Source: CAD feature listing. Evaluate the final solid. Frame: model axes, mm. A direction names the side the tool comes from. Give positions to 0.01 mm unless a question says otherwise; leave off trailing zeros. Write each loop counter-clockwise with the first axis right and the second up, starting at its lowest first coordinate (ties: lowest second). Pieces come first, ordered by that corner, then holes. Notation, with made-up numbers: (37.25, 77) -> (73.25, 77) arc R12 cw to (73.25, 98) -> close; hole circle Ø3 at (0, -37.5). An arc over 180 degrees is marked (long way). Use one line per item in the form item = value. Start each with the question number.
(1) Cut plane A-A, the plane z = 877. Output: boundary loops of the cut face in (x, y), and give its area (3 significant figures).
(2) Draft query along Z for faces 1 (the face through (71.048, -41.672, 776.376)), 2 (the face through (56, -61, 1574.8)), 3 (the face through (101.6, -169, 776)). Return one class per face: pulls with the +Z half, pulls with the -Z half, needs draft (parallel to the pull), parting line crosses it, or undercut.
(3) Material intervals for line 1 along Z through (x, y) = (8, -58); line 2 along Y through (x, z) = (25.4, 9.5); line 3 along X through (y, z) = (-198, 274), sorted ascending. Write a range as from..to.
(4) First-contact query: P1, Ø20.5, axis at x = 45.5, z = 8.5, coming from the -Y side; P2, Ø3, axis at x = 86, z = 1276.5, coming from the -Y side; P3, Ø5, axis at x = 13, z = 962, coming from the -Y side. Flat tips, straight axial feed; report the tip coordinate or a pass-through.
(5) Set-up query: faces 4 (the face through (114.3, -164, 776)), 5 (the face through (48, -88.032, 13)), 6 (the face through (48, -58, 25.4)). Return all of +Z, -Z, +X, -X, +Y, -Y with unobstructed straight access to the full face (end or side cutting, diameter ignored); none if empty.
from build123d import *

# Parameters (mm, degrees)
BOSS_EXTRUDE1_DEPTH = 1574.8
BOSS_EXTRUDE2_DEPTH = 25.4
SKETCH3_R           = 19.05
CUT_EXTRUDE1_DEPTH  = 1575.8


with BuildPart() as part:
    # Sketch1 → Boss-Extrude1 (new body)
    with BuildSketch(Plane.XY):
        with BuildLine():
            ThreePointArc((114.3, -101.6), (84.542048969, -29.757951031), (12.7, 0))
            ThreePointArc((12.7, 0), (6.337512086, -0.199414462), (0, -0.796875048))
            Line((0, -0.796875048), (0, -12.7))
            ThreePointArc((0, -12.7), (71.842048969, -42.457951031), (101.6, -114.3))
            Line((101.6, -114.3), (101.6, -224.550826558))
            Line((101.6, -224.550826558), (114.3, -224.550826558))
            Line((114.3, -224.550826558), (114.3, -101.6))
        make_face()
    extrude(amount=BOSS_EXTRUDE1_DEPTH)

    # Sketch2 → Boss-Extrude2 (add)
    with BuildSketch(Plane(origin=(0, 0, 0), x_dir=(-1, 0, 0), z_dir=(0, 0, -1))):
        with BuildLine():
            Line((0, -0.796875048), (0, -88.032487207))
            Line((0, -88.032487207), (-113.39003226, -88.032487207))
            ThreePointArc((-113.39003226, -88.032487207), (-74.652194888, -21.073696542), (0, -0.796875048))
        make_face()
    boss_extrude2 = extrude(amount=-BOSS_EXTRUDE2_DEPTH)

    # Mirror2: Boss-Extrude2 across plane
    add(boss_extrude2.mirror(Plane(origin=(0, 0, 787.4), x_dir=(1, 0, 0), z_dir=(0, 0, -1))))

    # Sketch3 → Cut-Extrude1 (cut, through all)
    with BuildSketch(Plane(origin=(0, 0, 0), x_dir=(-1, 0, 0), z_dir=(0, 0, -1))):
        with Locations((-25.4, -49.932487207)):
            Circle(SKETCH3_R)
    extrude(amount=-CUT_EXTRUDE1_DEPTH, mode=Mode.SUBTRACT)


solid = part.part
Geometry says:
q1.outline = (0, -12.7) arc R101.6 cw to (101.6, -114.3) -> (101.6, -224.55) -> (114.3, -224.55) -> (114.3, -101.6) arc R101.6 ccw to (0, -0.8) -> close
q1.area = 4,140 mm^2
q2.face_1 = undercut
q2.face_2 = pulls with the +Z half
q2.face_3 = needs draft
q3.line_1 = 0..25.4, 1549.4..1574.8
q3.line_2 = -88.03..-68.98, -30.88..-0.8
q3.line_3 = 101.6..114.3
q4.P1 = -88.03
q4.P2 = -62.66
q4.P3 = -13.89
q5.face_4 = +Z, -Z, +X, +Y, -Y
q5.face_5 = +Z, -Z, -X, -Y
q5.face_6 = -X, -Y
